The listing builds one solid part. Answer for the finished solid, in the listing's coordinates (mm). A direction names the side the tool comes from. Round coordinates to 2 decimals unless told otherwise and drop trailing zeros. Order: outer loops, then holes, each group sorted by start corner. A loop starts at its lowest first (then second) coordinate and runs counter-clockwise, first axis right, second up. Notation, with made-up numbers: (88.25, 84) -> (94.25, 84) arc R25 cw to (94.25, 121) -> close; hole circle Ø5 at (68.25, 9.5). An arc over 180 degrees is marked (long way). Return JSON: item names as keys, results as strings. Group by question number.
(1) The part is cut by section A-A (y = 0). Count the separate pieces of the cut face and the enclosed holes in it, plus the area to 3 significant figures.
(2) Which of the six approach directions +Z, -Z, +X, -X, +Y, -Y give full straight-line access (tool end or side, diameter ignored) to faces 4 (the face through (19, 3, 5)), 5 (the face through (26.846, -0.137, 1.972)), 6 (the face through (35.348, 0, 3))?
(3) Determine the mould class of faces 1 (the face through (19, 6.25, 2)), 2 (the face through (8.848, 0, 14)), 3 (the face through (0.85, 17.21, 13.58)) for opening direction Y: +Y half, -Y half, draft (parallel to the pull), parting line (faces both ways), or undercut.
(4) The part is cut by section C-C (x = 26). Determine the outline of the cut face in (y, z), plus the area to 3 significant figures.
(5) Consider line 1 (X direction, y = 0, z = 1.2); line 2 (Y direction, x = 20.5, z = 4.75); line 3 (Z direction, x = -30.5, y = -6.5). Determine where each line is inside the solid, lowest interval first. Write a range as [from, to].
(6) The part is cut by section B-B (x = -29). Determine the outline of the cut face in (y, z), plus the area to 3 significant figures.
(7) Each of these flat-tipped pins is pushed along its axis until it touches: pin 1 (15 mm diameter, centred on x = 19.5, y = -3, fed in from +Z); pin 2 (4.5 mm diameter, centred on x = -35.65, y = 0, fed in from -Z); pin 3 (1.5 mm diameter, centred on y = 3, z = 14, fed in from +X); pin 4 (5.5 mm diameter, centred on y = 3.5, z = 8.5, fed in from -X). Where does it stop, or does it pass through?
from build123d import *

# Parameters (mm, degrees)
F0_W            = 6
F0_H            = 35
F0_W_2          = 38.4963016563
F0_W_3          = 20.5
F1_DEPTH        = 6
F2_DEPTH        = 12
F3_SIZE         = 5
F4_DEPTH        = 21
F5_SIZE         = 5
F6_DEPTH        = 12
F7_T4_DEPTH     = 96.7203917112
F8_T1_DEPTH     = 35
F8_T3_DEPTH     = 28.0820880939
F8_T5_DEPTH     = 9.0857864376
F8_T7_DEPTH     = 9.1568542495
F8_T9_DEPTH     = 33
F8_T11_DEPTH    = 23.2989898732
F8_T13_DEPTH    = 37.0710678119
F8_T18_DEPTH    = 1.02
F8_T24_DEPTH    = 1.02
F8_T28_ANGLE    = 180
F8_T30_ANGLE    = 45
F8_T32_ANGLE    = 45
F9_R            = 0.8
F12_D           = 5
F12_CSINK_D     = 8.5
F12_CSINK_ANGLE = 90
F14_DEPTH       = 6
F15_DEPTH       = 4


# Not quite as in the source:
# - a fillet or chamfer that OpenCascade refuses, or shapes differently, is made with other operations: its cross-section is extruded or revolved along the edge and cut away or added


with BuildPart() as f1:
    # F0 (on Top) → F1 (new body)
    with BuildSketch(Plane.XY):
        with BuildLine():
            Line((-35.6485009767, -17.5), (-35.6485009767, 17.5))
            ThreePointArc((-35.6485009767, 17.5), (-53.1485009767, 0), (-35.6485009767, -17.5))
        make_face()
        with Locations((32.3478006796, 0)):
            Rectangle(F0_W, F0_H)
        with Locations((-16.4003501485, 0)):
            Rectangle(F0_W_2, F0_H)
        with Locations((19.0978006796, 0)):
            Rectangle(F0_W_3, F0_H)
        with Locations((5.8478006796, 0)):
            Rectangle(F0_W, F0_H)
    extrude(amount=F1_DEPTH)

    # F0 (on Top) → F2 (join)
    with BuildSketch(Plane.XY):
        with Locations((32.3478006796, 0)):
            Rectangle(F0_W, F0_H)
    extrude(amount=F2_DEPTH)

    # F3
    f3_edges = [f1.edges().sort_by_distance(p)[0] for p in [
        (35.347801, 0, 12),
    ]]
    chamfer(f3_edges, length=F3_SIZE)

    # F0 (on Top) → F4 (join)
    with BuildSketch(Plane.XY):
        with Locations((5.8478006796, 0)):
            Rectangle(F0_W, F0_H)
    extrude(amount=F4_DEPTH)

    # F5
    f5_edges = [f1.edges().sort_by_distance(p)[0] for p in [
        (2.847801, 0, 21),
    ]]
    chamfer(f5_edges, length=F5_SIZE)

    # F6 (add): a face of the model
    f6_faces = [f1.faces().sort_by_distance(p)[0] for p in [
        (2.8478006796, 0, 11),
    ]]
    extrude(f6_faces, amount=F6_DEPTH)

    # F7: chamfer of 12 on 4 edges, made by hand


with BuildPart() as f7_tool2:
    # F7_s3 → F7_t4 (new body)
    with BuildSketch(Plane.XZ.offset(-48.3601958556)):
        Polygon((2.8478006796, 16), (-9.1521993204, 4), (-9.1521993204, 16), align=None)
    extrude(amount=F7_T4_DEPTH)

    split(bisect_by=Plane.XY.offset(6), keep=Keep.TOP)


with BuildPart() as f1_1:
    add(f1.part)

    # F7_t1: cut F7_tool2
    add(f7_tool2.part, mode=Mode.SUBTRACT)

    # F8: fillet of radius 1 on 13 edges, made by hand

    # F8_s2 → F8_t1 (join)
    with BuildSketch(Plane.XZ.offset(-17.5)):
        with BuildLine():
            ThreePointArc((-7.5664128828, 6), (-7.1837294504, 6.0761204675), (-6.8593061016, 6.2928932188))
            Line((-6.8593061016, 6.2928932188), (-7.1521993204, 6))
            Line((-7.1521993204, 6), (-7.5664128828, 6))
        make_face()
    extrude(amount=F8_T1_DEPTH)

    # F8_s4 → F8_t3 (cut)
    with BuildSketch(Plane.YZ.offset(-35.6485009767)):
        with BuildLine():
            ThreePointArc((-16.5, 6), (-17.2071067812, 5.7071067812), (-17.5, 5))
            Line((-17.5, 5), (-17.5, 6))
            Line((-17.5, 6), (-16.5, 6))
        make_face()
        with BuildLine():
            ThreePointArc((17.5, 5), (17.2071067812, 5.7071067812), (16.5, 6))
            Line((16.5, 6), (17.5, 6))
            Line((17.5, 6), (17.5, 5))
        make_face()
    extrude(amount=F8_T3_DEPTH, mode=Mode.SUBTRACT)

    # F8_s6 → F8_t5 (cut)
    with BuildSketch(Plane.XY.offset(-2.5)):
        with BuildLine():
            ThreePointArc((35.3478006796, -16.5), (35.0549074608, -17.2071067812), (34.3478006796, -17.5))
            Line((34.3478006796, -17.5), (35.3478006796, -17.5))
            Line((35.3478006796, -17.5), (35.3478006796, -16.5))
        make_face()
        with BuildLine():
            ThreePointArc((34.3478006796, 17.5), (35.0549074608, 17.2071067812), (35.3478006796, 16.5))
            Line((35.3478006796, 16.5), (35.3478006796, 17.5))
            Line((35.3478006796, 17.5), (34.3478006796, 17.5))
        make_face()
    extrude(amount=F8_T5_DEPTH, mode=Mode.SUBTRACT)

    # F8_s8 → F8_t7 (cut)
    with BuildSketch(Plane(origin=(7.4061333868, 0, -7.4061333868), x_dir=(0, 1, 0), z_dir=(0.7071067812, 0, -0.7071067812))):
        with BuildLine():
            ThreePointArc((-16.5, 29.9444170289), (-17.2071067812, 29.6515238101), (-17.5, 28.9444170289))
            Line((-17.5, 28.9444170289), (-17.5, 29.9444170289))
            Line((-17.5, 29.9444170289), (-16.5, 29.9444170289))
        make_face()
        with BuildLine():
            ThreePointArc((17.5, 28.9444170289), (17.2071067812, 29.6515238101), (16.5, 29.9444170289))
            Line((16.5, 29.9444170289), (17.5, 29.9444170289))
            Line((17.5, 29.9444170289), (17.5, 28.9444170289))
        make_face()
    extrude(amount=F8_T7_DEPTH, mode=Mode.SUBTRACT)

    # F8_s10 → F8_t9 (cut)
    with BuildSketch(Plane.XZ.offset(-16.5)):
        with BuildLine():
            ThreePointArc((35.3478006796, 6.5857864376), (35.2716802121, 6.96846987), (35.0549074608, 7.2928932188))
            Line((35.0549074608, 7.2928932188), (35.3478006796, 7))
            Line((35.3478006796, 7), (35.3478006796, 6.5857864376))
        make_face()
    extrude(amount=F8_T9_DEPTH, mode=Mode.SUBTRACT)

    # F8_s12 → F8_t11 (cut)
    with BuildSketch(Plane(origin=(-0.2832064414, 0, -0.2832064414), x_dir=(0, 1, 0), z_dir=(0.7071067812, 0, 0.7071067812))):
        with BuildLine():
            ThreePointArc((17.5, 8.300009327), (17.2071067812, 9.0071161082), (16.5, 9.300009327))
            Line((16.5, 9.300009327), (17.5, 9.300009327))
            Line((17.5, 9.300009327), (17.5, 8.300009327))
        make_face()
        with BuildLine():
            ThreePointArc((-16.5, 9.300009327), (-17.2071067812, 9.0071161082), (-17.5, 8.300009327))
            Line((-17.5, 8.300009327), (-17.5, 9.300009327))
            Line((-17.5, 9.300009327), (-16.5, 9.300009327))
        make_face()
    extrude(amount=F8_T11_DEPTH, mode=Mode.SUBTRACT)

    # F8_s14 → F8_t13 (cut)
    with BuildSketch(Plane.XZ.offset(-18.5355339059)):
        with BuildLine():
            ThreePointArc((30.6406938984, 11.7071067812), (30.3162705496, 11.9238795325), (29.9335871172, 12))
            Line((29.9335871172, 12), (30.3478006796, 12))
            Line((30.3478006796, 12), (30.6406938984, 11.7071067812))
        make_face()
        with BuildLine():
            ThreePointArc((8.262014242, 21), (7.8793308096, 20.9238795325), (7.5549074608, 20.7071067812))
            Line((7.5549074608, 20.7071067812), (7.8478006796, 21))
            Line((7.8478006796, 21), (8.262014242, 21))
        make_face()
    extrude(amount=F8_T13_DEPTH, mode=Mode.SUBTRACT)


with BuildPart() as f8_tool16:
    # F8_s17 → F8_t18 (new body)
    with BuildSketch(Plane.XZ.offset(16.5)):
        Polygon((34.3478006796, 6.5857864376), (35.3678006796, 6.5857864376), (35.3678006796, 7.0082842712), (35.0690495964, 7.3070353544), align=None)
    extrude(amount=F8_T18_DEPTH)

    # F8_s19 → F8_t20 (revolve, cut)
    with BuildSketch(Plane(origin=(34.3478006796, -16.5, 6.5857864376), x_dir=(-0.9238795325, 0, -0.3826834324), z_dir=(-0.3826834324, 0, 0.9238795325))):
        with BuildLine():
            ThreePointArc((0, -1), (1, 0), (0, 1))
            Line((0, 1), (0, -1))
        make_face()
    revolve(axis=Axis((34.3478006796, -16.5, 6.5857864376), (0, -1, 0)), mode=Mode.SUBTRACT)


with BuildPart() as f1_2:
    add(f1_1.part)

    # F8_t15: cut F8_tool16
    add(f8_tool16.part, mode=Mode.SUBTRACT)


with BuildPart() as f8_tool22:
    # F8_s23 → F8_t24 (new body)
    with BuildSketch(Plane.XZ.offset(-16.5)):
        Polygon((34.3478006796, 6.5857864376), (35.3678006796, 6.5857864376), (35.3678006796, 7.0082842712), (35.0690495964, 7.3070353544), align=None)
    extrude(amount=-F8_T24_DEPTH)

    # F8_s25 → F8_t26 (revolve, cut)
    with BuildSketch(Plane(origin=(34.3478006796, 16.5, 6.5857864376), x_dir=(-0.9238795325, 0, -0.3826834324), z_dir=(0.3826834324, 0, -0.9238795325))):
        with BuildLine():
            ThreePointArc((0, -1), (1, 0), (0, 1))
            Line((0, 1), (0, -1))
        make_face()
    revolve(axis=Axis((34.3478006796, 16.5, 6.5857864376), (0, 1, 0)), mode=Mode.SUBTRACT)


with BuildPart() as f1_3:
    add(f1_2.part)

    # F8_t21: cut F8_tool22
    add(f8_tool22.part, mode=Mode.SUBTRACT)

    # F8_s27 → F8_t28 (revolve, cut)
    with BuildSketch(Plane.YZ.offset(-35.6485009767)):
        with BuildLine():
            ThreePointArc((16.5, 6), (17.2071067812, 5.7071067812), (17.5, 5))
            Line((17.5, 5), (17.5, 6))
            Line((17.5, 6), (16.5, 6))
        make_face()
    revolve(axis=Axis((-35.6485009767, 0, 6), (0, 0, 1)), revolution_arc=F8_T28_ANGLE, mode=Mode.SUBTRACT)

    # F8_s29 → F8_t30 (revolve, cut)
    with BuildSketch(Plane.YZ.offset(-7.5664128828)):
        with BuildLine():
            ThreePointArc((-17.5, 5), (-17.2071067812, 5.7071067812), (-16.5, 6))
            Line((-16.5, 6), (-17.5, 6))
            Line((-17.5, 6), (-17.5, 5))
        make_face()
    revolve(axis=Axis((-7.5664128828, -17.5, 7), (0, -1, 0)), revolution_arc=F8_T30_ANGLE, mode=Mode.SUBTRACT)

    # F8_s31 → F8_t32 (revolve, cut)
    with BuildSketch(Plane.YZ.offset(-7.5664128828)):
        with BuildLine():
            ThreePointArc((17.5, 5), (17.2071067812, 5.7071067812), (16.5, 6))
            Line((16.5, 6), (17.5, 6))
            Line((17.5, 6), (17.5, 5))
        make_face()
    revolve(axis=Axis((-7.5664128828, 17.5, 7), (0, -1, 0)), revolution_arc=F8_T32_ANGLE, mode=Mode.SUBTRACT)

    # F9
    f9_edges = [f1_3.edges().sort_by_distance(p)[0] for p in [
        (8.847801, 0, 6),
        (29.347801, 0, 6),
    ]]
    fillet(f9_edges, radius=F9_R)

    # F12 (through all)
    with Locations(Plane.XY.offset(6)):
        with Locations((-35.6485009767, 0)):
            CounterSinkHole(F12_D / 2, F12_CSINK_D / 2, counter_sink_angle=F12_CSINK_ANGLE)

    # F13 (on face) → F14 (cut, through all)
    with BuildSketch(Plane.XY):
        with BuildLine():
            ThreePointArc((20.5978006796, -3), (23.5978006796, 0), (20.5978006796, 3))
            Line((20.5978006796, 3), (17.5978006796, 3))
            ThreePointArc((17.5978006796, 3), (14.5978006796, 0), (17.5978006796, -3))
            Line((17.5978006796, -3), (20.5978006796, -3))
        make_face()
    extrude(amount=F14_DEPTH, mode=Mode.SUBTRACT)

    # F13 (on face) → F15 (cut)
    with BuildSketch(Plane.XY):
        with BuildLine():
            ThreePointArc((20.5978006796, -6.25), (26.8478006796, 0), (20.5978006796, 6.25))
            Line((20.5978006796, 6.25), (17.5978006796, 6.25))
            ThreePointArc((17.5978006796, 6.25), (11.3478006796, 0), (17.5978006796, -6.25))
            Line((17.5978006796, -6.25), (20.5978006796, -6.25))
        make_face()
        with BuildLine():
            Line((17.5978006796, 3), (20.5978006796, 3))
            ThreePointArc((20.5978006796, 3), (23.5978006796, 0), (20.5978006796, -3))
            Line((20.5978006796, -3), (17.5978006796, -3))
            ThreePointArc((17.5978006796, -3), (14.5978006796, 0), (17.5978006796, 3))
        make_face(mode=Mode.SUBTRACT)
    extrude(amount=F15_DEPTH, mode=Mode.SUBTRACT)


solid = f1_3.part
Answer below:
{
 "1": {"separate pieces": "3", "enclosed holes": "0", "area": "569 mm²"},
 "2": {"face 4": "+Z, -Z", "face 5": "-Z", "face 6": "+Z, -Z, +X, +Y, -Y"},
 "3": {"face 1": "undercut", "face 2": "draft", "face 3": "+Y half"},
 "4": {"outline": "(-17.5, 0) -> (-3.14, 0) -> (-3.14, 4) -> (3.14, 4) -> (3.14, 0) -> (17.5, 0) -> (17.5, 6) -> (-17.5, 6) -> close", "area": "185 mm²"},
 "5": {"line 1": "x = [-53.15, -38.15], [-33.15, 11.35], [26.85, 35.35]", "line 2": "y = [-17.5, -3], [3, 17.5]", "line 3": "z = [0, 6]"},
 "6": {"outline": "(-17.5, 0) -> (17.5, 0) -> (17.5, 5) arc R1 ccw to (16.5, 6) -> (-16.5, 6) arc R1 ccw to (-17.5, 5) -> close", "area": "210 mm²"},
 "7": {"pin 1": "stops at z = 6", "pin 2": "passes through", "pin 3": "stops at x = 8.85", "pin 4": "stops at x = -52.49"}
}
